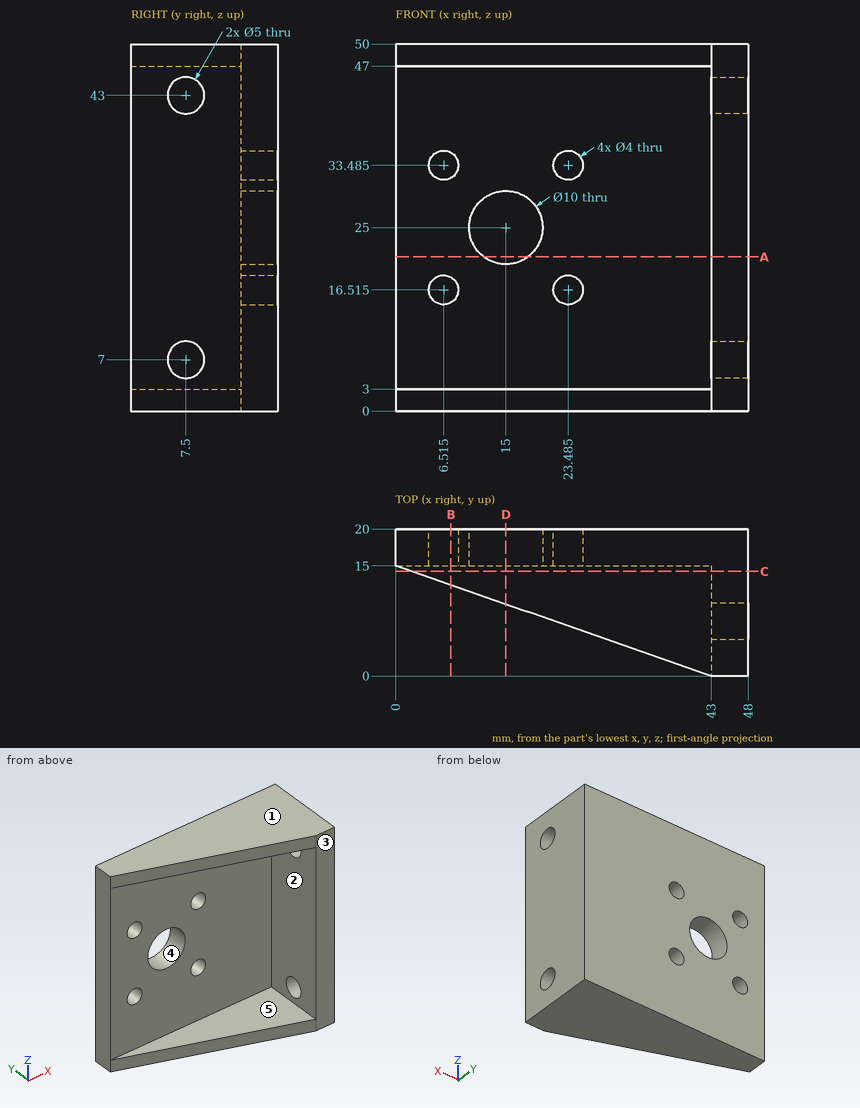
Answer from the drawing. Dimensions are ordinates in mm from the lowest x, y and z of the part. A direction names the side the tool comes from. Round coordinates to 2 decimals unless told otherwise and drop trailing zeros. Order: outer loops, then holes, each group sorted by start corner. A loop starts at its lowest first (then second) coordinate and runs counter-clockwise, first axis right, second up.
1) Flat-ended cylindrical pins translate along their axes: pin 1 (1.5 mm diameter, centred on y = 14, z = 44.5, fed in from -X); pin 2 (21.5 mm diameter, centred on x = 24.5, z = 23.5, fed in from -Y). Find the tip coordinate at first contact, or state that the pin passes through.
2) The mould has two halves that part along Z. Classify the marked faces 1, 2 and 3: released by +Z, released by -Z, zero draft, split by the parting line, or undercut.
3) The part is cut by section D-D on x = 15. Write down the section's boundary in (y, z).
4) For the marked faces 4 and 5, determine the directions among +Z, -Z, +X, -X, +Y, -Y from which every point of the face is accessible in a straight line to the end or side of a thin tool.
5) Straight lines are drawn through the part: L1, parallel to Z at x = 16.5, y = 10; L2, parallel to Y at x = 44.15, z = 43; L3, parallel to Y at x = 29.5, z = 22.5. For each, find the intervals that lie inside material, in ascending order.
6) The part is cut by section C-C on y = 14.25. Write down the section's boundary in (x, z).
7) The part is cut by section B-B on x = 7.5. Write down the section's boundary in (y, z) (1 decimal), plus the area to 3 significant figures.
8) The part is cut by section A-A on z = 21. Write down the section's boundary in (x, y), plus the area to 3 significant figures.
Resolved:
1. pin 1: stops at x = 43
1. pin 2: stops at y = 15
2. face 1: released by +Z
2. face 2: undercut
2. face 3: zero draft
3. outline: (9.77, 0) - (20, 0) - (20, 20) - (15, 20) - (15, 3) - (9.77, 3) - close; (9.77, 47) - (15, 47) - (15, 30) - (20, 30) - (20, 50) - (9.77, 50) - close
4. face 4: +Y, -Y
4. face 5: -X, -Y
5. L1: z = 0 to 3, 47 to 50
5. L2: y = 0 to 5, 10 to 20
5. L3: y = 15 to 20
6. outline: (2.15, 0) - (48, 0) - (48, 50) - (2.15, 50) - (2.15, 47) - (43, 47) - (43, 3) - (2.15, 3) - close
7. outline: (12.4, 0) - (20, 0) - (20, 14.8) - (15, 14.8) - (15, 3) - (12.4, 3) - close; (12.4, 47) - (15, 47) - (15, 35.2) - (20, 35.2) - (20, 50) - (12.4, 50) - close; (15, 18.3) - (20, 18.3) - (20, 31.7) - (15, 31.7) - close
7. area: 231 mm2
8. outline: (0, 15) - (12, 15) - (12, 20) - (0, 20) - close; (18, 15) - (43, 15) - (43, 0) - (48, 0) - (48, 20) - (18, 20) - close
8. area: 285 mm2
